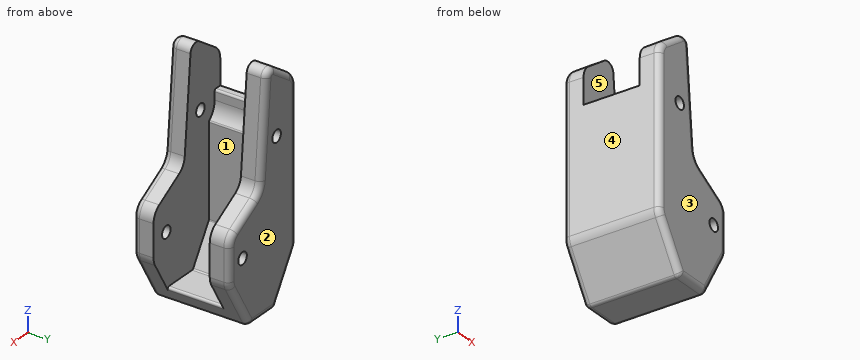
```python
from build123d import *

# Parameters (mm, degrees)
SKETCH036_R     = 1.5
PAD021_DEPTH    = 24
FILLET007_R     = 1.5
POCKET013_DEPTH = 14
FILLET008_R     = 0.5


with BuildPart() as part:
    # Sketch036 → Pad021 (new body)
    with BuildSketch(Plane.XZ):
        with BuildLine():
            Line((-59.294306, 24.684125), (-53.647153, 28.638304))
            ThreePointArc((-50.507611, 27.174311), (-51.654763, 28.812616), (-53.647153, 28.638304))
            Line((-50.507611, 27.174311), (-48.491026, 4.124639))
            ThreePointArc((-48.491026, 4.124639), (-47.879813, 2.324063), (-46.506247, 1.00916))
            Line((-39.5, -3.035898), (-46.506247, 1.00916))
            ThreePointArc((-37.5, -6.5), (-38.035898, -4.5), (-39.5, -3.035898))
            Line((-37.5, -6.5), (-37.5, -14.5))
            ThreePointArc((-38.041032, -16.508866), (-37.637626, -15.540223), (-37.5, -14.5))
            Line((-38.041032, -16.508866), (-44.135258, -27.002216))
            ThreePointArc((-45, -27.5), (-44.501109, -27.366665), (-44.135258, -27.002216))
            Line((-45, -27.5), (-53, -27.5))
            ThreePointArc((-53.846615, -27.032205), (-53.483629, -27.375273), (-53, -27.5))
            Line((-53.846615, -27.032205), (-60.386462, -16.628821))
            ThreePointArc((-61, -14.5), (-60.843556, -15.607735), (-60.386462, -16.628821))
            Line((-61, -14.5), (-61, 21.407517))
            ThreePointArc((-59.294306, 24.684125), (-60.548043, 23.254511), (-61, 21.407517))
        make_face()
        with Locations((-54, 12.5)):
            Circle(SKETCH036_R, mode=Mode.SUBTRACT)
        with Locations((-42, -10.5)):
            Circle(SKETCH036_R, mode=Mode.SUBTRACT)
    extrude(amount=PAD021_DEPTH)

    # Fillet007
    fillet007_edges = [part.edges().sort_by_distance(p)[0] for p in [
        (-60.548043, 0, 23.254511),
        (-60.548043, -24, 23.254511),
    ]]
    fillet(fillet007_edges, radius=FILLET007_R)

    # Sketch037 (on Face12 of Fillet007) → Pocket013 (cut)
    with BuildSketch(Plane.XZ.offset(19)):
        with BuildLine():
            Line((-37.475618, -23.5), (-51.342359, -23.5))
            Line((-51.342359, -23.5), (-57, -14.5))
            Line((-57, -14.5), (-57, 8.5))
            ThreePointArc((-59, 12.5), (-58.472136, 10.263932), (-57, 8.5))
            Line((-59, 12.5), (-59, 15))
            Line((-59, 15), (-79, 15))
            Line((-79, 15), (-79, 35))
            Line((-79, 35), (-15.733307, 35))
            Line((-15.733307, 35), (-15.733307, -20.5))
            Line((-15.733307, -20.5), (-35.733307, -20.5))
            Line((-35.733307, -20.5), (-37.475618, -23.5))
        make_face()
    extrude(amount=-POCKET013_DEPTH, mode=Mode.SUBTRACT)

    # Fillet008
    fillet008_edges = [part.edges().sort_by_distance(p)[0] for p in [
        (-57, -12, 8.5),
        (-59, -12, 15),
        (-57, -12, -14.5),
        (-51.342359, -12, -23.5),
        (-42.101275, -12, -23.5),
    ]]
    fillet(fillet008_edges, radius=FILLET008_R)


with BuildPart() as part_1:
    # Body003 placement: moved
    add(part.part.moved(Location((0, 33, 0))))


with BuildPart() as part_2:
    # Clone170 placement: moved
    add(part_1.part.moved(Location((-47, -47, 7.5))))


solid = part_2.part
```
Geometry: final body of the model. Coordinates: model frame, mm. Face numbers are marked on the shaded views. A direction names the side the tool comes from. Coordinates: 2 decimals unless noted, no trailing zeros. Order: outer loops, then holes, each group sorted by start corner. A loop starts at its lowest first (then second) coordinate and runs counter-clockwise, first axis right, second up.
Item 1: Access query for the marked faces 1 and 2. Directions: +Z, -Z, +X, -X, +Y, -Y. A direction counts if a zero-diameter tool reaches every point of the face in a straight line with its end or side. Return the directions, or none.
Answer:
face 1: +Z, +X
face 2: +Z, -Z, +X, -X, +Y
Item 2: Section query A-A (z = -3). Output: boundary loops of the cut face in (x, y).
Answer:
outline: (-108, -36.5) arc R1.5 ccw to (-106.5, -38) - (-90.5, -38) - (-90.5, -33) - (-104, -33) - (-104, -19) - (-90.5, -19) - (-90.5, -14) - (-106.5, -14) arc R1.5 ccw to (-108, -15.5) - close; (-87.5, -38) - (-86, -38) arc R1.5 ccw to (-84.5, -36.5) - (-84.5, -33) - (-87.5, -33) - close; (-87.5, -19) - (-84.5, -19) - (-84.5, -15.5) arc R1.5 ccw to (-86, -14) - (-87.5, -14) - close
Item 3: Section query B-B (x = -101.5). State how many separate pieces and enclosed holes the cut face has, then the cut area to 3 significant figures.
Answer:
separate pieces: 3
enclosed holes: 0
area: 614 mm2
Item 4: Draft query along Y for the marked faces 3, 4 and 5. Return one class per face: released by +Y, released by -Y, zero draft, split by the parting line, or undercut.
Answer:
face 3: released by -Y
face 4: zero draft
face 5: undercut
Item 5: Contact query for flat-ended pins moving along their axis: P1, Ø0.6, axis at y = -25.5, z = 21, coming from the +X side; P2, Ø9, axis at x = -95, y = -24.5, coming from the +Z side; P3, Ø11, axis at y = -25.5, z = 3, coming from the +X side. Output: stop coordinate, or through.
Answer:
P1: stops at x = -106
P2: stops at z = -14.16
P3: stops at x = -104
Item 6: Material intervals for line 1 along Y through (x, z) = (-97.75, -14); line 2 along X through (y, z) = (-35.7, -3); line 3 along X through (y, z) = (-23.5, 8.5), sorted ascending.
Answer:
line 1: y = -38 to -33, -19 to -14
line 2: x = -108 to -90.5, -87.5 to -84.5
line 3: x = -108 to -104
Item 7: Section query C-C (y = -25.5). Output: boundary loops of the cut face in (x, z).
Answer:
outline: (-108, -7) arc R4 ccw to (-107.39, -9.13) - (-100.85, -19.53) arc R1 ccw to (-100, -20) - (-92, -20) arc R1 ccw to (-91.14, -19.5) - (-89.54, -16.75) arc R0.5 ccw to (-89.97, -16) - (-98.07, -16) arc R0.5 cw to (-98.49, -15.77) - (-103.92, -7.12) arc R0.5 cw to (-104, -6.86) - (-104, 15.76) arc R0.5 ccw to (-104.18, 16.14) arc R5 cw to (-106, 20) - (-106, 22) arc R0.5 ccw to (-106.5, 22.5) - (-108, 22.5) - close
